Autodesk Inventor part; units mm, degrees
ref_plane "PLANE RH" through (457.2, 0, 0) normal (1, 0, 0) x (0, 1, 0)
ref_plane "PLANE LH" through (-457.2, 0, 0) normal (1, 0, 0) x (0, 1, 0)
ref_plane "PLANE BOT" through (0, 0, -203.2) normal (0, 0, 1) x (1, 0, 0)
ref_plane "PLANE IN" through (0, 0, 0) normal (0, 1, 0) x (-1, 0, 0)
ref_plane "PLANE OUT" through (0, 1524, 0) normal (0, 1, 0) x (-1, 0, 0)
ref_plane "PLANE CTR" through (0, 0, 0) normal (1, 0, 0) x (0, 1, 0)
ref_plane "PLANE RH" through (457.2, 0, 0) normal (1, 0, 0) x (0, 1, 0)
ref_plane "PLANE LH" through (-457.2, 0, 0) normal (1, 0, 0) x (0, 1, 0)
ref_plane "PLANE TOP" through (0, 0, 0) normal (0, 0, 1) x (1, 0, 0)
ref_plane "PLANE BOT" through (0, 0, -203.2) normal (0, 0, 1) x (1, 0, 0)
ref_plane "PLANE HANDLE RH" through (558.8, 0, 0) normal (1, 0, 0) x (0, 1, 0)
ref_plane "PLANE HANDLE LH" through (-558.8, 0, 0) normal (1, 0, 0) x (0, 1, 0)
ref_plane "PLANE HANDLE IN" through (0, 63.5, 0) normal (0, 1, 0) x (-1, 0, 0)
ref_plane "PLANE HANDLE OUT" through (0, 1460.5, 0) normal (0, 1, 0) x (-1, 0, 0)
ref_plane "PLANE HANDLE TOP" through (0, 0, -63.5) normal (0, 0, 1) x (1, 0, 0)
sketch "SKETCH BODY" plane through (0, 0, 0) normal (0, 0, 1) x (1, 0, 0)
  line L0 (-457.2, 0) -> (457.2, 0)
  line L1 (457.2, 0) -> (457.2, 1524)
  line L2 (457.2, 1524) -> (-457.2, 1524)
  line L3 (-457.2, 1524) -> (-457.2, 0)
  line L4 (-640.08, 0) -> (640.08, 0)
  line L5 (-640.08, 1524) -> (640.08, 1524)
  line L6 (457.2, 3657.6) -> (457.2, -609.6)
  line L7 (-457.2, 3657.6) -> (-457.2, -609.6)
extrude "EXT BODY" add sketch "SKETCH BODY" against normal blind 203.2
sketch "SKETCH HANDLE DIA" plane through (457.2, 0, 0) normal (1, 0, 0) x (0, 1, 0)
  line L0 (45.72, -63.5) -> (81.28, -63.5)
  line L1 (63.5, -45.72) -> (63.5, -81.28)
  circle A0 centre (63.5, -63.5) radius 12.7
  dimension "d79" = 25.4
sketch "SKETCH HANDLE PATH" plane through (0, 0, -63.5) normal (0, 0, 1) x (1, 0, 0)
  line L0 (558.8, 3568.7) -> (558.8, -520.7)
  line L1 (457.2, 3568.7) -> (457.2, -520.7)
  line L2 (436.88, 63.5) -> (579.12, 63.5)
  line L3 (436.88, 1460.5) -> (579.12, 1460.5)
  line L4 (457.2, 63.5) -> (558.8, 63.5)
  line L5 (558.8, 63.5) -> (558.8, 1460.5)
  line L6 (558.8, 1460.5) -> (457.2, 1460.5)
  line L7 (457.2, 1460.5) -> (457.2, 63.5) construction
sweep "SWP HANDLE" add profiles "SKETCH HANDLE DIA" path "SKETCH HANDLE PATH" path curves L4 L5 L6
mirror "MIR HANDLE" about plane through (0, 0, 0) normal (1, 0, 0)
equation "\"d76\" = HEIGHT"
equation "\"PLANE_OUT\" = LENGTH"
equation "\"PLANE_RH\" = 0.5 * WIDTH"
equation "\"PLANE_LH\" = -0.5 * WIDTH"
equation "\"PLANE_BOT\" = -HEIGHT"
equation "\"PLANE_HANDLE_RH\" = HANDLE_OFFSET_CTR"
equation "\"PLANE_HANDLE_LH\" = -HANDLE_OFFSET_CTR"
equation "\"PLANE_HANDLE_IN\" = HANDLE_OFFSET_END"
equation "\"PLANE_HANDLE_OUT\" = LENGTH - HANDLE_OFFSET_END"
equation "\"PLANE_HANDLE_TOP\" = -HANDLE_OFFSET_TOP"
equation "\"LENGTH\" = 1524"
equation "\"WIDTH\" = 914.4"
equation "\"HEIGHT\" = 203.2"
equation "\"HANDLE_GAP\" = 101.6"
equation "\"HANDLE_OFFSET_CTR\" = 0.5 * WIDTH + HANDLE_GAP"
equation "\"HANDLE_OFFSET_END\" = 63.5"
equation "\"HANDLE_OFFSET_TOP\" = 63.5"
properties part number "ATQ-36-60-B"
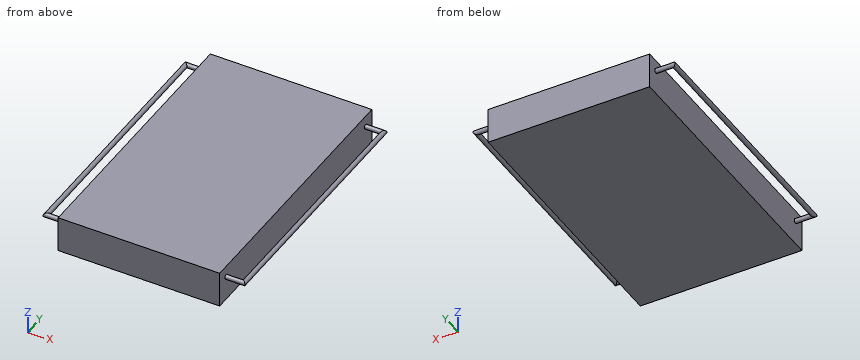
Verification items for the finished model (mm, model axes). Give positions to 0.01 mm unless a question says otherwise; leave off trailing zeros. Loops run counter-clockwise (first coordinate to the right, second up) from the corner with the lowest first, then second, coordinate; pieces in that order, holes last.
1. Material ranges on probe 1 along X at (y, z) = (986, -56); probe 2 along X at (y, z) = (958.5, -172), recorded low to high.
Derived:
probe 1: x = -569.05 to -548.55, -457.2 to 457.2, 548.55 to 569.05
probe 2: x = -457.2 to 457.2
2. Cross-section at A-A on y = 683. Record the cut outline in (x, z).
Derived:
outline: circle Ø25.4 at (-558.8, -63.5); (-457.2, -203.2) - (457.2, -203.2) - (457.2, 0) - (-457.2, 0) - close; circle Ø25.4 at (558.8, -63.5)
3. Go/stop test with flat-tipped pins: P1, Ø10, axis at y = 1195, z = -123.5, coming from the -X side; P2, Ø8, axis at y = 521.5, z = -76, coming from the -X side; P3, Ø3, axis at y = 819.5, z = -76.5, coming from the +X side. Record where each tip stops, or that it passes through.
Derived:
P1: stops at x = -457.2
P2: stops at x = -568.24
P3: stops at x = 564.19
4. Cross-section at B-B on z = -160.5. Record the cut outline in (x, y).
Derived:
outline: (-457.2, 0) - (457.2, 0) - (457.2, 1524) - (-457.2, 1524) - close
